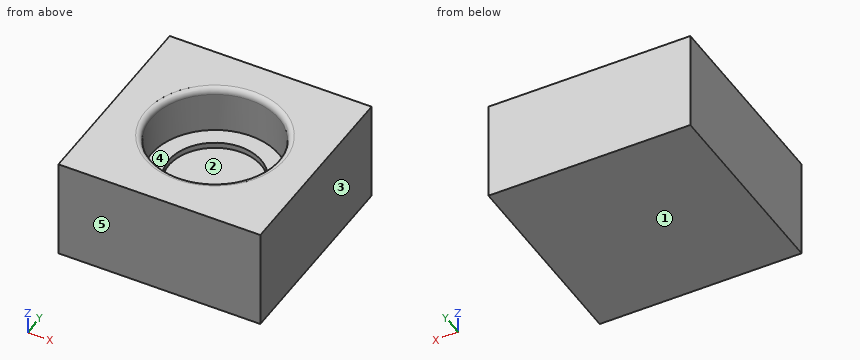
Autodesk Fusion 360 part; units mm, degrees
sketch "Sketch2" plane through (0, 0, 0) normal (0, 0, 1) x (1, 0, 0)
  line L0 (17.5, 17.5) -> (-17.5, 17.5)
  line L1 (-17.5, 17.5) -> (-17.5, -17.5)
  line L2 (-17.5, -17.5) -> (17.5, -17.5)
  line L3 (17.5, -17.5) -> (17.5, 17.5)
  line L4 (17.5, 17.5) -> (-17.5, -17.5) construction
  line L5 (-17.5, 17.5) -> (17.5, -17.5) construction
  dimension "d10" = 35
  dimension "d11" = 35
extrude "Extrude2" add sketch "Sketch2" along normal blind 17.5
sketch "Sketch3" plane through (0, 0, 17.5) normal (0, 0, 1) x (-1, 0, 0)
  line L0 (-17.5, 17.5) -> (-17.5, -17.5)
  line L1 (-17.5, -17.5) -> (17.5, -17.5)
  line L2 (17.5, -17.5) -> (17.5, 17.5)
  line L3 (17.5, 17.5) -> (-17.5, 17.5)
  circle A0 centre (0, 0) radius 11.05
  dimension "d14" = 22.1
extrude "Extrude3" cut sketch "Sketch3" against normal blind 8 contours A0
sketch "Sketch4" plane through (0, 0, 9.5) normal (0, 0, 1) x (-1, 0, 0)
  circle A0 centre (0, 0) radius 11.05
  circle A1 centre (0, 0) radius 8
  dimension "d20" = 16
extrude "Extrude4" cut sketch "Sketch4" against normal blind 1 contours A1
sketch "Sketch5" plane through (0, 0, 8.5) normal (0, 0, 1) x (-1, 0, 0)
  circle A0 centre (0, 0) radius 8
  circle A1 centre (0, 0) radius 5
  dimension "d23" = 10
extrude "Extrude5" cut sketch "Sketch5" along normal through all contours A1
fillet "Fillet1" radius 1 1 edges at (10.3022, -3.9959, 17.5)
equation "TOL = 0.1 mm"
equation "BlockSize = 35 mm"
equation "d10 = BlockSize"
equation "d11 = BlockSize"
equation "d12 = BlockSize / 2"
equation "d14 = BearingOuter + TOL"
equation "d15 = -( BearingDepth + 1 mm )"
equation "BearingOuter = 22 mm"
equation "BearingInner = 8 mm"
equation "BearingWall = 2 mm"
equation "d20 = BearingOuter - BearingWall * 3"
equation "d23 = BearingInner + 2 mm"
equation "BearingDepth = 7 mm"
The model under review builds one solid part; all positions refer to its coordinate system, in mm. Face numbers are marked on the shaded views. A direction names the side the tool comes from. Round coordinates to 2 decimals unless told otherwise and drop trailing zeros. Loops run counter-clockwise (first coordinate to the right, second up) from the corner with the lowest first, then second, coordinate; pieces in that order, holes last. Notation, with made-up numbers: M 72.5,65 L 106.5,65 A22 ccw 106.5,78 Z; hole C 52.5,68 d4. An arc over 180 degrees is marked long. Answer as a JSON object with one key per item and string values.
Item 1: Clearance check with flat-ended pins moving along their axes: P1, Ø13, axis at x = 3.5, y = 2, coming from the +Z side; P2, Ø21, axis at x = 0, y = 0, coming from the -Z side; P3, Ø13.5, axis at x = 0, y = 0, coming from the +Z side. State where each tip first meets the part, or that it passes through.
Check sheet entries:
{"P1": "z = 9.5", "P2": "z = 0", "P3": "z = 8.5"}
Item 2: We need section C-C, the plane z = 12.75. State the section outline as (x, y) points, and give its area (3 significant figures).
Check sheet entries:
{"outline": "M -17.5,-17.5 L 17.5,-17.5 L 17.5,17.5 L -17.5,17.5 Z; hole C 0,0 d22.1", "area": "841 mm2"}
Item 3: Tool access review of the marked faces 1 and 2: name each direction out of +Z, -Z, +X, -X, +Y, -Y from which nothing blocks a thin tool from reaching the whole face with its end or side.
Check sheet entries:
{"face 1": "-Z, +X, -X, +Y, -Y", "face 2": "+Z"}
Item 4: The part is to be moulded in two halves that separate along X. For the marked faces 3, 4 and 5, say which applies: +X half, -X half, draft (parallel to the pull), parting line (faces both ways), or undercut.
Check sheet entries:
{"face 3": "+X half", "face 4": "undercut", "face 5": "draft"}
Item 5: For line 1 along X through (y, z) = (0, 8.8); line 2 along X through (y, z) = (0, 11.5), list the stretches that pass through material, from the lowest coordinate up.
Check sheet entries:
{"line 1": "-17.5 to -8, 8 to 17.5", "line 2": "-17.5 to -11.05, 11.05 to 17.5"}
Item 6: We need section A-A, the plane x = 0. State the section outline as (y, z) points.
Check sheet entries:
{"outline": "M -17.5,0 L 17.5,0 L 17.5,17.5 L 12.05,17.5 A1 ccw 11.05,16.5 L 11.05,9.5 L 8,9.5 L 8,8.5 L -8,8.5 L -8,9.5 L -11.05,9.5 L -11.05,16.5 A1 ccw -12.05,17.5 L -17.5,17.5 Z"}
